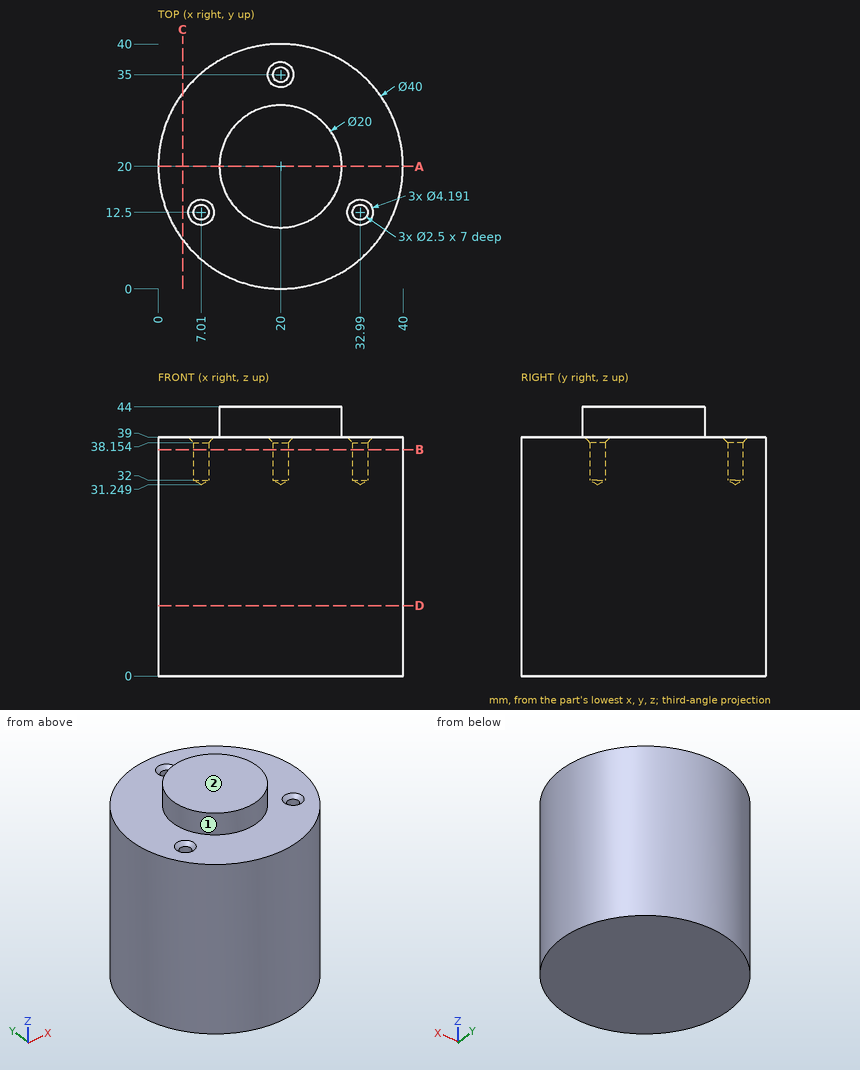
Print and shaded views of the part. All mm, measured from the part's lowest x, y and z. A direction names the side the tool comes from. Coordinates: 2 decimals unless noted, no trailing zeros. Order: outer loops, then holes, each group sorted by start corner. A loop starts at its lowest first (then second) coordinate and runs counter-clockwise, first axis right, second up. Notation, with made-up numbers: M 38.5,6.5 L 63.5,6.5 A6 ccw 63.5,11.5 Z; hole C -33.75,-16.5 d10. An arc over 180 degrees is marked long. Answer as CSV lines item,"result".
1) Drill centre lines: L1, parallel to Z at x = 19, y = 3.5; L2, parallel to X at y = 12.5, z = 35; L3, parallel to X at y = 12, z = 35 (1 decimal). Where is each one in solid material? Low to high. Write a range as from..to.
Verdict:
L1,"0..39"
L2,"1.46..5.76, 8.26..31.74, 34.24..38.54"
L3,"1.7..5.9, 8.2..31.8, 34.1..38.3"
2) Flat gauge pins, fed straight in: P1, Ø1, axis at x = 16, y = 23, coming from the -Z side; P2, Ø1.5, axis at x = 30, z = 32.5, coming from the -Y side; P3, Ø1.5, axis at x = 32.99, y = 12.5, coming from the +Z side; P4, Ø4, axis at y = 6, z = 17.5, coming from the -X side. Where does each tip first touch, or does it go through?
Verdict:
P1,"z = 0"
P2,"y = 2.27"
P3,"z = 31.7"
P4,"x = 4"
3) 3-axis set-ups, long thin cutter, end or side, ignore diameter. For the marked faces 1 and 2: which of +Z, -Z, +X, -X, +Y, -Y reach the whole face in a straight line?
Verdict:
face 1,"+Z"
face 2,"+Z, +X, -X, +Y, -Y"
4) Cut at A-A (y = 20). List the corners of the cut face in (x, z), then the cut area to 3 significant figures.
Verdict:
outline,"M 0,0 L 40,0 L 40,39 L 30,39 L 30,44 L 10,44 L 10,39 L 0,39 Z"
area,"1,660 mm2"
5) Cut at B-B (z = 37). List the corners of the cut face in (x, y).
Verdict:
outline,"C 20,20 d40; hole C 7.01,12.5 d2.5; hole C 20,35 d2.5; hole C 32.99,12.5 d2.5"
6) Cut at D-D (z = 11.5). List the corners of the cut face in (x, y).
Verdict:
outline,"C 20,20 d40"
7) Cut at C-C (x = 4). List the corners of the cut face in (y, z), then the cut area to 3 significant figures.
Verdict:
outline,"M 8,0 L 32,0 L 32,39 L 8,39 Z"
area,"936 mm2"
